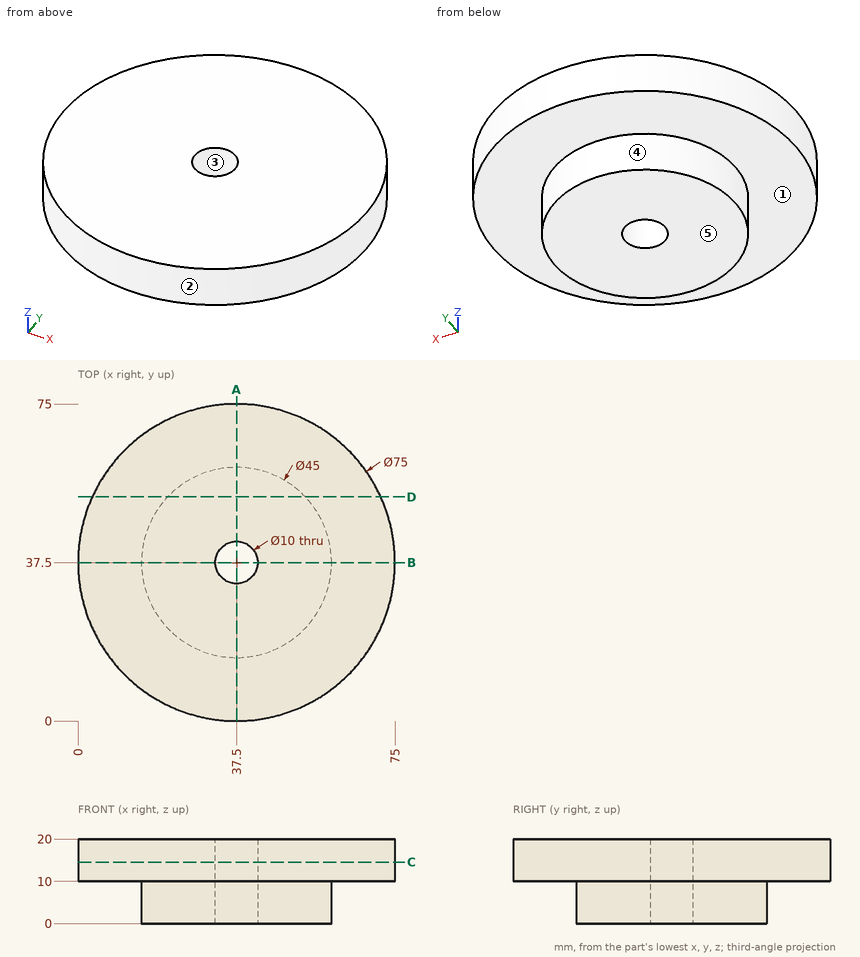
Check sheet for the drawn part. Datum: minimum x, y, z corner. Units: mm. A direction names the side the tool comes from. Coordinates: 2 decimals unless noted, no trailing zeros. Order: outer loops, then holes, each group sorted by start corner. A loop starts at its lowest first (then second) coordinate and runs counter-clockwise, first axis right, second up. Notation, with made-up numbers: M 14,79 L 38,79 A18 cw 38,83 Z; hole C 78.5,-20.75 d2. An arc over 180 degrees is marked long. One line per item, written item: value. Start each with the question number.
Item 1: Mould release check, pull along Y, two halves, no side actions. Record for the marked faces 3, 4 and 5: released by +Y, released by -Y, zero draft, split by the parting line, or undercut.
Item 2: Sectioned sample at A-A (x = 37.5). Enter the section's corners in (y, z).
Item 3: Sectioned sample at C-C (z = 14.5). Enter the section's corners in (x, y), then the cut area to 3 significant figures.
Item 4: Sectioned sample at D-D (y = 53). Enter the section's corners in (x, z), then the cut area to 3 significant figures.
Item 5: Scan lines: probe 1 along Y at (x, z) = (37.5, 13); probe 2 along Z at (x, y) = (57, 22.5); probe 3 along Y at (x, z) = (37.5, 6.5). Record each from-to range of solid material in increasing order.
Item 6: Gauge pin test, flat ends, axial feed: pin 1 (1.5 mm diameter, centred on y = 35, z = 8, fed in from +X); pin 2 (6 mm diameter, centred on y = 65.5, z = 15.5, fed in from -X); pin 3 (5 mm diameter, centred on y = 44.5, z = 3.5, fed in from +X). Record the tip position at first contact, or that the pin passes through.
Item 7: Access from +Z, -Z, +X, -X, +Y, -Y to the whole of each face (thin tool, end or side, straight path). Record for the marked faces 1 and 2.
Conclusion:
1. face 3: undercut
1. face 4: split by the parting line
1. face 5: zero draft
2. outline: M 0,10 L 15,10 L 15,0 L 32.5,0 L 32.5,20 L 0,20 Z; M 42.5,0 L 60,0 L 60,10 L 75,10 L 75,20 L 42.5,20 Z
3. outline: C 37.5,37.5 d75; hole C 37.5,37.5 d10
3. area: 4,340 mm^2
4. outline: M 3.35,10 L 21.19,10 L 21.19,0 L 53.81,0 L 53.81,10 L 71.65,10 L 71.65,20 L 3.35,20 Z
4. area: 1,010 mm^2
5. probe 1: y = 0 to 32.5, 42.5 to 75
5. probe 2: z = 10 to 20
5. probe 3: y = 15 to 32.5, 42.5 to 60
6. pin 1: stops at x = 59.93
6. pin 2: stops at x = 9.55
6. pin 3: stops at x = 59.55
7. face 1: -Z
7. face 2: +Z, -Z
